Model file for the job. Use its own axes, mm. Face numbers are marked on the shaded views. A direction names the side the tool comes from. Round coordinates to 2 decimals unless told otherwise and drop trailing zeros. Order: outer loops, then holes, each group sorted by start corner. A loop starts at its lowest first (then second) coordinate and runs counter-clockwise, first axis right, second up. Notation, with made-up numbers: (74.25, -3.5) -> (78.25, -3.5) arc R18 ccw to (78.25, 15.5) -> close; hole circle Ø5 at (20.25, 84.25). An arc over 180 degrees is marked (long way). Put each result on its own line as item: value. Start each with the question number.
Q1. Flat gauge pins, fed straight in: P1, Ø2, axis at x = 4, y = 6, coming from the +Z side; P2, Ø2.5, axis at x = -2, z = -9, coming from the +Y side; P3, Ø3.5, axis at x = -0.5, y = -2, coming from the +Z side; P4, Ø5.5, axis at x = 0, z = 8.5, coming from the -Y side. Where does each tip first touch, or does it go through?
Q2. Cut at C-C, the plane y = 8.75. List the corners of the cut face in (x, z).
Q3. Pull direction X, two halves, no side cores. Call the marked faces 6, 7, 8 and 9: released by +X, released by -X, zero draft, split by the parting line, or undercut.
Q4. Cut at B-B, the plane z = 8.5. List the corners of the cut face in (x, y), and give its area (3 significant figures).
Q5. Cut at A-A, the plane x = 0. List the corners of the cut face in (y, z), and give its area (3 significant figures).
Q6. Cut at D-D, the plane z = -8. List the corners of the cut face in (x, y).
Q7. 3-axis set-ups, long thin cutter, end or side, ignore diameter. For the marked faces 1, 2, 3, 4 and 5: which of +Z, -Z, +X, -X, +Y, -Y reach the whole face in a straight line?
Q8. Probe L1, parallel to X at y = 5, z = -8; L2, parallel to X at y = 3.75, z = 7.75; L3, parallel to Z at x = 7.5, y = 8.75. List the from-to ranges inside material, lowest first.
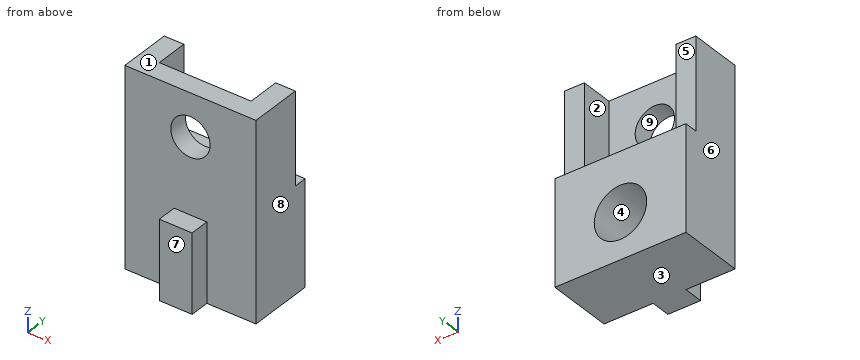
from build123d import *

# Parameters (mm, degrees)
SKETCH1_W               = 20
SKETCH1_H               = 30
BOSS_EXTRUDE1_DEPTH     = 3
SKETCH2_W               = 5
SKETCH2_H               = 12
BOSS_EXTRUDE2_DEPTH     = 3
SKETCH3_R               = 7
SKETCH3_R_2             = 4
BOSS_EXTRUDE3_DEPTH     = 7
SKETCH4_R               = 4
BOSS_EXTRUDE4_DEPTH     = 1
CUT_EXTRUDE1_DEPTH      = 20.339079606
CUT_EXTRUDE1_DEPTH_BACK = 20.339079606
SKETCH5_R               = 3
SKETCH6_R               = 7
SKETCH6_R_2             = 4
BOSS_EXTRUDE6_DEPTH     = 7
SKETCH7_W               = 20
SKETCH7_H               = 3
BOSS_EXTRUDE7_DEPTH     = 19
SKETCH8_W               = 5
SKETCH8_H               = 3
BOSS_EXTRUDE8_DEPTH     = 12
CUT_EXTRUDE2_START      = -1.5
SKETCH10_R              = 4
CUT_EXTRUDE2_DEPTH      = 1.5
SKETCH12_W              = 3
SKETCH12_H              = 32
BOSS_EXTRUDE9_DEPTH     = 5
CUT_EXTRUDE3_DEPTH      = 52
CUT_EXTRUDE3_DEPTH_BACK = 52
SKETCH13_W              = 44.018077629
SKETCH13_H              = 41.98282258
CUT_EXTRUDE4_DEPTH      = 2


with BuildPart() as part:
    # Sketch1 → Boss-Extrude1 (new body)
    with BuildSketch(Plane(origin=(0, 0, 0), x_dir=(1, 0, 0), z_dir=(0, 1, 0))):
        Rectangle(SKETCH1_W, SKETCH1_H)
    boss_extrude1 = extrude(amount=BOSS_EXTRUDE1_DEPTH)

    # Sketch2 → Boss-Extrude2 (add)
    with BuildSketch(Plane.XZ):
        with Locations((0, -9)):
            Rectangle(SKETCH2_W, SKETCH2_H)
    boss_extrude2 = extrude(amount=BOSS_EXTRUDE2_DEPTH)

    # Sketch3 → Boss-Extrude3 (add)
    with BuildSketch(Plane(origin=(0, 3, 0), x_dir=(1, 0, 0), z_dir=(0, 1, 0))):
        with Locations(Location((0, 8, 0), (0, 0, 90))):
            Circle(SKETCH3_R)
        with Locations(Location((0, 8, 0), (0, 0, 270))):
            Circle(SKETCH3_R_2, mode=Mode.SUBTRACT)
    boss_extrude3 = extrude(amount=BOSS_EXTRUDE3_DEPTH)

    # Sketch4 → Boss-Extrude4 (add)
    with BuildSketch(Plane(origin=(0, 3, 0), x_dir=(1, 0, 0), z_dir=(0, 1, 0))):
        with Locations(Location((0, 8, 0), (0, 0, 270))):
            Circle(SKETCH4_R)
    boss_extrude4 = extrude(amount=BOSS_EXTRUDE4_DEPTH)

    # Sketch5 → Cut-Extrude1 (cut, two sides: drawn at the far end of the back side and taken through both)
    with BuildSketch(Plane(origin=(0, 3, 0), x_dir=(1, 0, 0), z_dir=(0, 1, 0)).offset(-CUT_EXTRUDE1_DEPTH_BACK)):
        with Locations(Location((0, -8.5, 0), (0, 0, 90))):
            Circle(SKETCH5_R)
    extrude(amount=CUT_EXTRUDE1_DEPTH + CUT_EXTRUDE1_DEPTH_BACK, mode=Mode.SUBTRACT)

    # Sketch6 → Boss-Extrude6 (add)
    # profile 1 of 2: a face of its own
    with BuildSketch(Plane(origin=(0, 3, 0), x_dir=(1, 0, 0), z_dir=(0, 1, 0))):
        Polygon((0, 15), (-10, 15), (-10, -1), (10, -1), (10, 15), align=None)
        with BuildLine():
            ThreePointArc((7, 8), (-4.949747468, 3.050252532), (0, 15))
            ThreePointArc((0, 15), (4.949747468, 12.949747468), (7, 8))
        make_face(mode=Mode.SUBTRACT)
    # profile 2 of 2: a face of its own
    with BuildSketch(Plane(origin=(0, 3, 0), x_dir=(1, 0, 0), z_dir=(0, 1, 0))):
        with Locations((0, 8)):
            Circle(SKETCH6_R)
        with Locations(Location((0, 8, 0), (0, 0, 270))):
            Circle(SKETCH6_R_2, mode=Mode.SUBTRACT)
    boss_extrude6 = extrude(amount=BOSS_EXTRUDE6_DEPTH)

    # Sketch7 → Boss-Extrude7 (add)
    with BuildSketch(Plane.XY.offset(15)):
        with Locations((0, 1.5)):
            Rectangle(SKETCH7_W, SKETCH7_H)
    extrude(amount=BOSS_EXTRUDE7_DEPTH)

    # Mirror3: Boss-Extrude1, Boss-Extrude2, Boss-Extrude3, Boss-Extrude4, Boss-Extrude6 across plane
    add(boss_extrude1.mirror(Plane.XY.offset(17)))
    add(boss_extrude2.mirror(Plane.XY.offset(17)))
    add(boss_extrude3.mirror(Plane.XY.offset(17)))
    add(boss_extrude4.mirror(Plane.XY.offset(17)))
    add(boss_extrude6.mirror(Plane.XY.offset(17)))

    # Sketch8 → Boss-Extrude8 (add)
    with BuildSketch(Plane(origin=(0, 0, 37), x_dir=(-1, 0, 0), z_dir=(0, 0, -1))):
        with Locations((0, -1.5)):
            Rectangle(SKETCH8_W, SKETCH8_H)
    extrude(amount=BOSS_EXTRUDE8_DEPTH)

    # Sketch10 → Cut-Extrude2 (cut)
    with BuildSketch(Plane(origin=(0, 4, 0), x_dir=(1, 0, 0), z_dir=(0, 1, 0)).offset(CUT_EXTRUDE2_START)):
        with Locations(Location((0, 8, 0), (0, 0, 270))):
            Circle(SKETCH10_R)
        with Locations(Location((0, -42, 0), (0, 0, 90))):
            Circle(SKETCH10_R)
    extrude(amount=CUT_EXTRUDE2_DEPTH, mode=Mode.SUBTRACT)

    # Sketch12 → Boss-Extrude9 (add)
    with BuildSketch(Plane(origin=(0, 3, 0), x_dir=(1, 0, 0), z_dir=(0, 1, 0))):
        with Locations((8.5, -17)):
            Rectangle(SKETCH12_W, SKETCH12_H)
        with Locations((-8.5, -17)):
            Rectangle(SKETCH12_W, SKETCH12_H)
    extrude(amount=BOSS_EXTRUDE9_DEPTH)

    # Sketch13 → Cut-Extrude3 (cut, two sides: drawn at the far end of the back side and taken through both)
    with BuildSketch(Plane(origin=(0, 0, 0), x_dir=(1, 0, 0), z_dir=(0, 1, 0)).offset(-CUT_EXTRUDE3_DEPTH_BACK)):
        with Locations((-0.328555997, -37.99141129)):
            Rectangle(SKETCH13_W, SKETCH13_H)
    extrude(amount=CUT_EXTRUDE3_DEPTH + CUT_EXTRUDE3_DEPTH_BACK, mode=Mode.SUBTRACT)

    # Sketch14 → Cut-Extrude4 (cut)
    with BuildSketch(Plane.XY.offset(17)):
        Polygon((10, 8), (7, 8), (7, 3), (-7, 3), (-7, 8), (-10, 8), (-10, 0), (10, 0), align=None)
    extrude(amount=-CUT_EXTRUDE4_DEPTH, mode=Mode.SUBTRACT)


solid = part.part
Ans:
1. P1: stops at z = 1
1. P2: stops at y = 2.5
1. P3: stops at z = -3
1. P4: passes through
2. outline: (-10, -15) -> (10, -15) -> (10, 1) -> (-10, 1) -> close; hole circle Ø8 at (0, -8)
3. face 6: released by -X
3. face 7: zero draft
3. face 8: released by +X
3. face 9: undercut
4. outline: (-10, 0) -> (-3, 0) -> (-3, 3) -> (-7, 3) -> (-7, 8) -> (-10, 8) -> close; (3, 0) -> (10, 0) -> (10, 8) -> (7, 8) -> (7, 3) -> (3, 3) -> close
4. area: 72.0 mm^2
5. outline: (-3, -15) -> (10, -15) -> (10, -12) -> (2.5, -12) -> (2.5, -4) -> (10, -4) -> (10, 1) -> (3, 1) -> (3, 5.5) -> (0, 5.5) -> (0, -3) -> (-3, -3) -> close; (0, 11.5) -> (3, 11.5) -> (3, 15) -> (0, 15) -> close
5. area: 160 mm^2
6. outline: (-10, 0) -> (-2.5, 0) -> (-2.5, -3) -> (2.5, -3) -> (2.5, 0) -> (10, 0) -> (10, 10) -> (4, 10) -> (4, 2.5) -> (-4, 2.5) -> (-4, 10) -> (-10, 10) -> close
7. face 1: +Z, +X, -X, +Y, -Y
7. face 2: +Z, +Y
7. face 3: -Z, +X, -X, +Y, -Y
7. face 4: +Y
7. face 5: +Z, +X, -X, +Y
8. L1: x = -10 to -4, 4 to 10
8. L2: x = -10 to -7, 7 to 10
8. L3: z = -15 to 1
